Could you check a few things on this model? Use its own coordinates, in mm. Round coordinates to 2 decimals unless told otherwise and drop trailing zeros. Loops run counter-clockwise (first coordinate to the right, second up) from the corner with the lowest first, then second, coordinate; pieces in that order, holes last. Notation, with made-up numbers: (88.25, 4) - (114.25, 4) arc R20 ccw to (114.25, 40) - close; hole circle Ø3 at (36, 39). An arc over 180 degrees is marked (long way). Use one line per item in the form item = value.
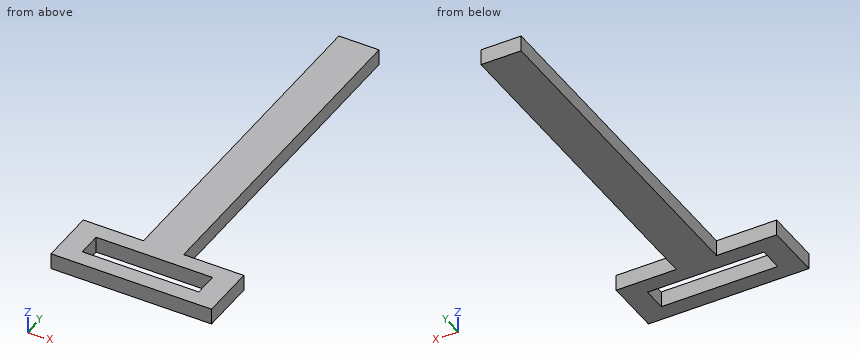
```python
from build123d import *

# Parameters (mm, degrees)
BOX002_W     = 5
BOX002_H     = 42.400002
BOX002_DEPTH = 2
BOX001_W     = 14.5
BOX001_H     = 3
BOX001_DEPTH = 2
BOX_W        = 20
BOX_H        = 7
BOX_DEPTH    = 2


with BuildPart() as box002:
    # Box002 → Box002 (new body)
    with BuildSketch(Plane(origin=(7.5, 7, 0), x_dir=(1, 0, 0), z_dir=(0, 0, 1))):
        with Locations((2.5, 21.200001)):
            Rectangle(BOX002_W, BOX002_H)
    extrude(amount=BOX002_DEPTH)


with BuildPart() as box001:
    # Box001 → Box001 (new body)
    with BuildSketch(Plane(origin=(2.75, 2, 0), x_dir=(1, 0, 0), z_dir=(0, 0, 1))):
        with Locations((7.25, 1.5)):
            Rectangle(BOX001_W, BOX001_H)
    extrude(amount=BOX001_DEPTH)


with BuildPart() as fusion:
    # Box → Box (new body)
    with BuildSketch(Plane.XY):
        with Locations((10, 3.5)):
            Rectangle(BOX_W, BOX_H)
    extrude(amount=BOX_DEPTH)

    # Cut: cut Box001
    add(box001.part, mode=Mode.SUBTRACT)

    # Fusion: union Box002
    add(box002.part)


solid = fusion.part
```
1. If we section it at D-D, the plane y = 44: Write out the boundary of the cut face in (x, z), plus the area to 3 significant figures.
Solution:
outline = (7.5, 0) - (12.5, 0) - (12.5, 2) - (7.5, 2) - close
area = 10.0 mm^2
2. If we section it at C-C, the plane z = 0.5: Write out the boundary of the cut face in (x, y).
Solution:
outline = (0, 0) - (20, 0) - (20, 7) - (12.5, 7) - (12.5, 49.4) - (7.5, 49.4) - (7.5, 7) - (0, 7) - close; hole (2.75, 2) - (17.25, 2) - (17.25, 5) - (2.75, 5) - close
3. Please list where these lines run through material, in increasing order: line 1 along Y through (x, z) = (15, 0.4); line 2 along Y through (x, z) = (10.25, 1.25); line 3 along X through (y, z) = (25.5, 0.6).
Solution:
line_1 = 0 to 2, 5 to 7
line_2 = 0 to 2, 5 to 49.4
line_3 = 7.5 to 12.5
4. If we section it at B-B, the plane x = 11.75: Write out the boundary of the cut face in (y, z).
Solution:
outline = (0, 0) - (2, 0) - (2, 2) - (0, 2) - close; (5, 0) - (49.4, 0) - (49.4, 2) - (5, 2) - close
5. If we section it at A-A, the plane y = 4: Write out the boundary of the cut face in (x, z).
Solution:
outline = (0, 0) - (2.75, 0) - (2.75, 2) - (0, 2) - close; (17.25, 0) - (20, 0) - (20, 2) - (17.25, 2) - close
